Part model, mm, in its own coordinate system. Face numbers are marked on the shaded views. A direction names the side the tool comes from. Give positions to 0.01 mm unless a question says otherwise; leave off trailing zeros. Loops run counter-clockwise (first coordinate to the right, second up) from the corner with the lowest first, then second, coordinate; pieces in that order, holes last. Notation, with made-up numbers: (24.5, 60.25) -> (46.5, 60.25) arc R29 cw to (46.5, 90.25) -> close; hole circle Ø7 at (53, -36.5). An arc over 180 degrees is marked (long way). One line per question, with ' | ' between items.
Autodesk Inventor part; units mm, degrees
ref_plane "YZ Plane" through (0, 0, 0) normal (1, 0, 0) x (0, 1, 0)
ref_plane "XZ Plane" through (0, 0, 0) normal (0, 1, 0) x (-1, 0, 0)
ref_plane "XY Plane" through (0, 0, 0) normal (0, 0, 1) x (1, 0, 0)
ref_plane "작업 평면1" through (0, 0, 0) normal (0, 0, 1) x (1, 0, 0)
sketch "스케치1" plane through (0, 0, 0) normal (0, 0, 1) x (1, 0, 0)
  circle A0 centre (-7.7782, -7.7782) radius 1.55
  circle A1 centre (7.7782, -7.7782) radius 1.55
  circle A2 centre (7.7782, 7.7782) radius 1.55
  circle A3 centre (-7.7782, 7.7782) radius 1.55
  circle A4 centre (0, 0) radius 5
  circle A5 centre (0, 11) radius 1.55
  circle A6 centre (11, 0) radius 1.55
  circle A7 centre (0, -11) radius 1.55
  circle A8 centre (-11, 0) radius 1.55
  circle A9 centre (0, 0) radius 5.1
  line L0 (-13.9, 0) -> (13.9, 0)
  line L1 (13.9, 0) -> (13.9, 13.9)
  line L2 (13.9, 13.9) -> (-13.9, 13.9)
  line L3 (-13.9, 13.9) -> (-13.9, 0)
  line L4 (-5.1, 0) -> (-5.1, -12.9306)
  line L5 (5.1, 0) -> (5.1, -12.9306)
  circle A10 centre (-7.7782, 7.7782) radius 1.6
  circle A11 centre (-11, 0) radius 1.6
  circle A12 centre (-7.7782, -7.7782) radius 1.6
  circle A13 centre (0, -11) radius 1.6
  circle A14 centre (7.7782, -7.7782) radius 1.6
  circle A15 centre (11, 0) radius 1.6
  circle A16 centre (7.7782, 7.7782) radius 1.6
  circle A17 centre (0, 11) radius 1.6
  line L6 (-13.9, 13.9) -> (13.9, 13.9)
  circle A18 centre (-7.7782, -7.7782) radius 1.55
  circle A19 centre (7.7782, -7.7782) radius 1.55
  circle A20 centre (7.7782, 7.7782) radius 1.55
  circle A21 centre (-7.7782, 7.7782) radius 1.55
  circle A22 centre (0, 0) radius 5
  circle A23 centre (0, 0) radius 13.9
  circle A24 centre (0, 11) radius 1.55
  circle A25 centre (11, 0) radius 1.55
  circle A26 centre (0, -11) radius 1.55
  circle A27 centre (-11, 0) radius 1.55
  circle A28 centre (0, 0) radius 13.9
  line L7 (-13.9, 13.9) -> (13.9, 13.9)
  line L8 (13.9, 13.9) -> (13.9, 40.9)
  line L9 (13.9, 40.9) -> (-13.9, 40.9)
  line L10 (-13.9, 40.9) -> (-13.9, 13.9)
  dimension "d0" = 0.1
  dimension "d1" = 3.2
  dimension "d4" = 360
  dimension "d10" = 27
  dimension "d16" = 13.9
extrude "돌출4" add sketch "스케치1" along normal blind 6 contours A9 L0 A11 A23 A15 | L0 A15 A23 L5 | L4 A23 L0 A11 | A23 L2 L1 | L3 L2 A23 | L2 L10 L9 L8
mirror "미러4" about plane through (13.9, 40.9, 0) normal (0, 1, 0)
fillet "모깎기3" radius 2 4 edges at (5.1, 94.7306, 3) (-5.1, 94.7306, 3) (5.1, -12.9306, 3) (-5.1, -12.9306, 3)
properties part number "leg_ver2_new" material "PMMA 플라스틱"
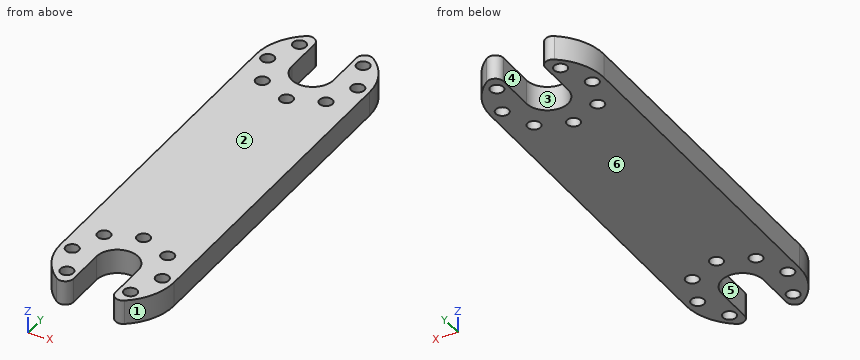
1) Saw through at B-B (y = 11). Give the cut face in (x, z), and give its area (3 significant figures).
Found:
outline: (-13.9, 0) -> (-1.6, 0) -> (-1.6, 6) -> (-13.9, 6) -> close; (1.6, 0) -> (13.9, 0) -> (13.9, 6) -> (1.6, 6) -> close | area: 148 mm2
2) Saw through at A-A (x = 0). Give the cut face in (y, z), and give its area (3 significant figures).
Found:
outline: (5.1, 0) -> (9.4, 0) -> (9.4, 6) -> (5.1, 6) -> close; (12.6, 0) -> (69.2, 0) -> (69.2, 6) -> (12.6, 6) -> close; (72.4, 0) -> (76.7, 0) -> (76.7, 6) -> (72.4, 6) -> close | area: 391 mm2
3) Drill centre lines: line 1 (X direction, y = 0, z = 2.25); line 2 (Y direction, x = -10.75, z = 3.25); line 3 (X direction, y = 7, z = 5.05). Where is each one in solid material? Low to high.
Found:
line 1: -13.9 to -12.6, -9.4 to -5.1, 5.1 to 9.4, 12.6 to 13.9 | line 2: -8.81 to -1.58, 1.58 to 80.22, 83.38 to 90.61 | line 3: -13.9 to -9.18, -6.38 to 6.38, 9.18 to 13.9
4) Saw through at D-D (x = -11). Give the cut face in (y, z), and give its area (3 significant figures).
Found:
outline: (-8.5, 0) -> (-1.6, 0) -> (-1.6, 6) -> (-8.5, 6) -> close; (1.6, 0) -> (80.2, 0) -> (80.2, 6) -> (1.6, 6) -> close; (83.4, 0) -> (90.3, 0) -> (90.3, 6) -> (83.4, 6) -> close | area: 554 mm2
5) Pin check, flat tips, straight feed: P1, Ø1.5, axis at x = -2.5, y = 48.5, coming from the -Z side; P2, Ø1.5, axis at x = -2, z = 4, coming from the -Y side; P3, Ø3, axis at x = 0, z = 3, coming from the +Y side. Stop position of each tip, or through.
Found:
P1: z = 0 | P2: y = 4.3 | P3: y = 76.93
6) Tool access for the marked faces 4, 5 and 6: list every direction of +Z, -Z, +X, -X, +Y, -Y with a clear straight run to the whole face (end or side of a thin tool).
Found:
face 4: +Z, -Z, +Y | face 5: +Z, -Z, -Y | face 6: -Z, +X, -X, +Y, -Y
7) Pull direction X, two halves, no side cores. Call the marked faces 1, 2 and 3: pulls with the +X half, pulls with the -X half, needs draft (parallel to the pull), parting line crosses it, or undercut.
Found:
face 1: pulls with the +X half | face 2: needs draft | face 3: undercut
8) Saw through at C-C (z = 1.65). State how many separate pieces and enclosed holes the cut face has, and give its area (3 significant figures).
Found:
separate pieces: 1 | enclosed holes: 14 | area: 2,400 mm2
